Design review of the part shown in the three views and the two pictorial views. Dimensions are in mm from the part's minimum x, y and z. A direction names the side the tool comes from. Give positions to 0.01 mm unless a question says otherwise; leave off trailing zeros. Order: outer loops, then holes, each group sorted by start corner. A loop starts at its lowest first (then second) coordinate and runs counter-clockwise, first axis right, second up. Notation, with made-up numbers: (-37.5, 55.5) - (-4.5, 55.5) arc R16 ccw to (-4.5, 79.5) - close; hole circle Ø5 at (-15, -5.5). An arc over 180 degrees is marked (long way). Put each result on its own line as item: value.
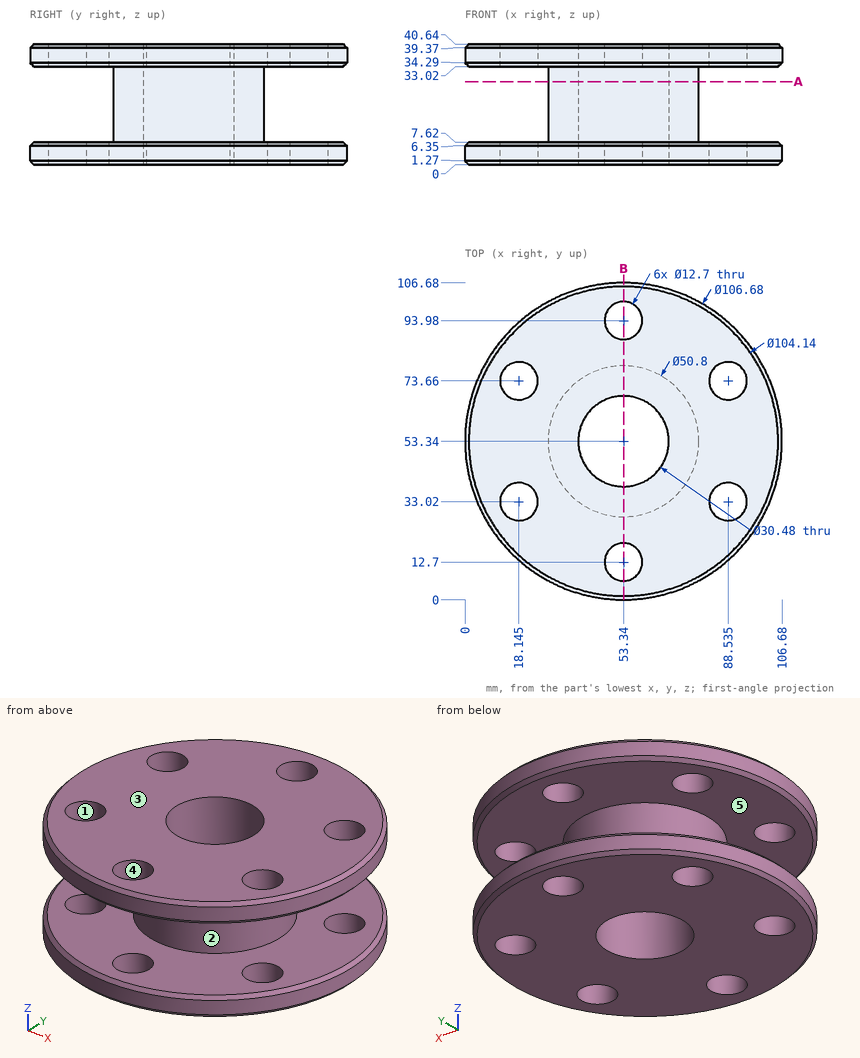
(1) The part is to be moulded in two halves that separate along Z. For the marked faces 3, 4 and 5, say which applies: pulls with the +Z half, pulls with the -Z half, needs draft (parallel to the pull), parting line crosses it, or undercut.
The answers:
face 3: pulls with the +Z half
face 4: needs draft
face 5: undercut
(2) Take a section at A-A, the plane z = 28. Write out the cut boundary in (x, y).
The answers:
outline: circle Ø50.8 at (53.34, 53.34); hole circle Ø30.48 at (53.34, 53.34)
(3) Wall thickness on L1, parallel to Z at x = 8, y = 44.5; L2, parallel to X at y = 31.5, z = 5; L3, parallel to Y at x = 16, z = 34 (1 decimal): over which ranges is each line inside the solid? List them lowest first.
The answers:
L1: 0 to 7.62, 33.02 to 40.64
L2: 4.68 to 11.98, 24.31 to 82.37, 94.7 to 102
L3: 15.7 to 27, 39 to 67.7, 79.6 to 91
(4) For the marked faces 1 and 2, list the 3-axis set-ups (+Z, -Z, +X, -X, +Y, -Y) from which the entire face can be reached by the end or side of a thin tool; tool diameter is ignored.
The answers:
face 1: +Z, -Z
face 2: none
(5) Clearance check with flat-ended pins moving along their axes: pin 1 Ø2 at (y, z) = (37.5, 34) entering from +X; pin 2 Ø11.5 at (x, y) = (88.54, 33.02) entering from -Z; pin 3 Ø5 at (y, z) = (29.5, 24) entering from -X (1 decimal); pin 4 Ø3 at (y, z) = (47.5, 22) entering from -X. State where each tip first meets the part, or that it passes through.
The answers:
pin 1: x = 104.56
pin 2: through
pin 3: x = 39.6
pin 4: x = 28.31
(6) Take a section at B-B, the plane x = 53.34. Count the separate pieces of the cut face and the enclosed holes in it, then the cut area to 3 significant figures.
The answers:
separate pieces: 6
enclosed holes: 0
area: 1,280 mm^2
